Can you work these out from the drawing? Everything is in mm from the part's minimum corner. A direction names the side the tool comes from. Coordinates: 2 decimals unless noted, no trailing zeros. Write each loop counter-clockwise with the first axis right and the second up, starting at its lowest first coordinate (ties: lowest second). Pieces come first, ordered by that corner, then holes.
(1) Thinking about a two-plate mould opening in Y: for the marked faces 4, 5, 6 and 7, which applies, released by +Y, released by -Y, zero draft, split by the parting line, or undercut?
(2) Please list where these lines run through material, in increasing order: probe 1 along Y at (x, z) = (10.75, 16); probe 2 along Y at (x, z) = (23.5, 3); probe 3 along X at (y, z) = (8.25, 8).
(3) Imagine slicing it at C-C, the plane y = 11.5. List the corners of the cut face in (x, z) for me.
(4) Imagine slicing it at B-B, the plane x = 9.5. List the corners of the cut face in (y, z) for me.
(5) Imagine slicing it at D-D, the plane z = 3. List the corners of the cut face in (x, y) for me.
(6) For pin 1 Ø4.5 at (x, y) = (3.5, 5) entering from -Z; pin 2 Ø6.5 at (x, y) = (4.5, 5.5) entering from +Z; pin 3 Ø3.5 at (x, y) = (23.5, 20) entering from +Z, each with a flat end and sliding along its axis, tell me the tip position at first contact or that it passes through.
(7) Which directions (+Z, -Z, +X, -X, +Y, -Y) give clear straight access to the entire face, cutting with the end or side of a thin tool? Please do the marked faces 1, 2 and 3.
(8) Imagine slicing it at A-A, the plane z = 16. List the corners of the cut face in (x, y) for me, plus the area to 3 significant figures.
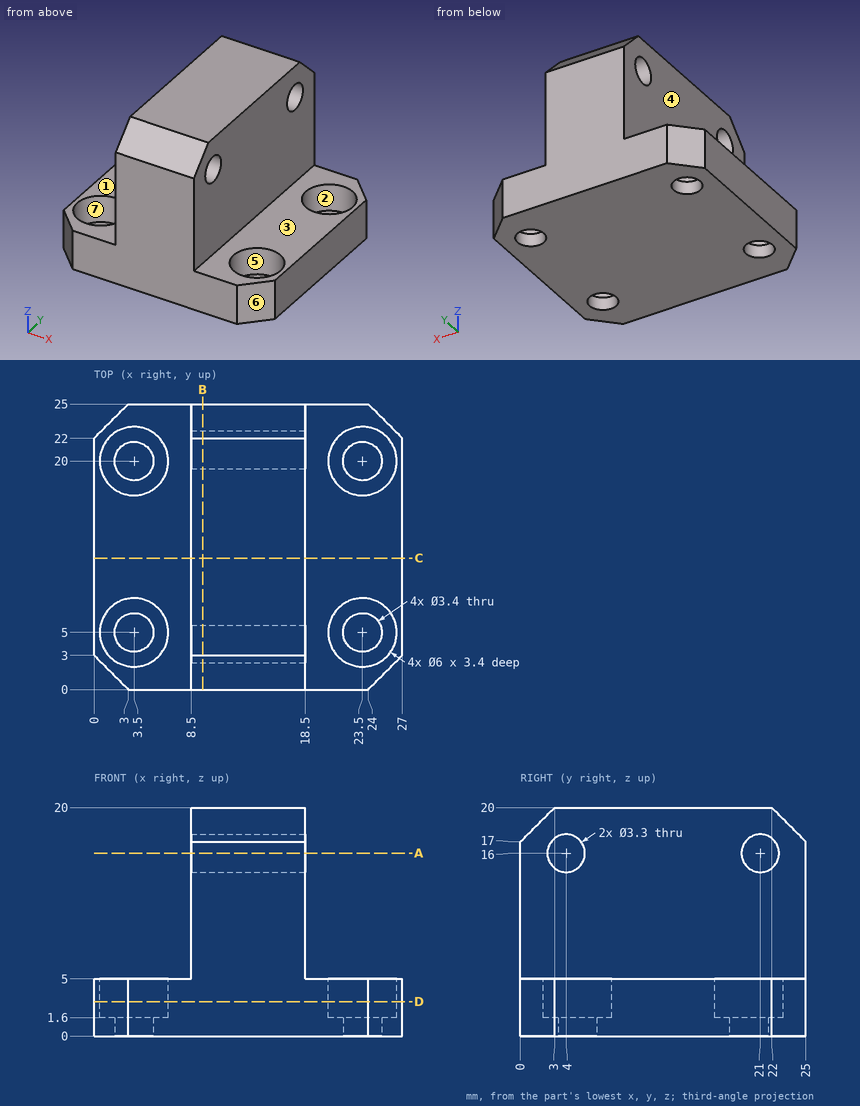
Recorded:
1. face 4: zero draft
1. face 5: undercut
1. face 6: released by -Y
1. face 7: undercut
2. probe 1: y = 0 to 2.35, 5.65 to 19.35, 22.65 to 25
2. probe 2: y = 0 to 2, 8 to 17, 23 to 25
2. probe 3: x = 8.5 to 18.5
3. outline: (0, 0) - (27, 0) - (27, 5) - (18.5, 5) - (18.5, 20) - (8.5, 20) - (8.5, 5) - (0, 5) - close
4. outline: (0, 0) - (25, 0) - (25, 17) - (22, 20) - (3, 20) - (0, 17) - close; hole circle Ø3.3 at (4, 16); hole circle Ø3.3 at (21, 16)
5. outline: (0, 3) - (3, 0) - (24, 0) - (27, 3) - (27, 22) - (24, 25) - (3, 25) - (0, 22) - close; hole circle Ø6 at (3.5, 5); hole circle Ø6 at (3.5, 20); hole circle Ø6 at (23.5, 5); hole circle Ø6 at (23.5, 20)
6. pin 1: stops at z = 0
6. pin 2: stops at z = 5
6. pin 3: stops at z = 1.6
7. face 1: +Z, -X, +Y, -Y
7. face 2: +Z
7. face 3: +Z, +X, +Y, -Y
8. outline: (8.5, 0) - (18.5, 0) - (18.5, 2.35) - (8.5, 2.35) - close; (8.5, 5.65) - (18.5, 5.65) - (18.5, 19.35) - (8.5, 19.35) - close; (8.5, 22.65) - (18.5, 22.65) - (18.5, 25) - (8.5, 25) - close
8. area: 184 mm2
